from build123d import *

# Parameters (mm, degrees)
SKETCH1_R           = 1.5
BOSS_EXTRUDE1_DEPTH = 7
SKETCH2_R           = 1.4
BOSS_EXTRUDE2_DEPTH = 0.5
BOSS_EXTRUDE3_START = 0.5
SKETCH3_R           = 1.5
BOSS_EXTRUDE3_DEPTH = 0.5


with BuildPart() as part:
    # Sketch1 → Boss-Extrude1 (new body)
    with BuildSketch(Plane.XY):
        Circle(SKETCH1_R)
    extrude(amount=BOSS_EXTRUDE1_DEPTH)

    # Sketch2 → Boss-Extrude2 (add)
    with BuildSketch(Plane(origin=(0, 0, 0), x_dir=(-1, 0, 0), z_dir=(0, 0, -1))):
        Circle(SKETCH2_R)
    boss_extrude2 = extrude(amount=BOSS_EXTRUDE2_DEPTH)

    # Sketch3 → Boss-Extrude3 (add)
    with BuildSketch(Plane(origin=(0, 0, -0.5), x_dir=(-1, 0, 0), z_dir=(0, 0, -1)).offset(BOSS_EXTRUDE3_START)):
        with Locations(Location((0, 0, 0), (0, 0, 180))):
            Circle(SKETCH3_R)
    boss_extrude3 = extrude(amount=-BOSS_EXTRUDE3_DEPTH)

    # Mirror1: Boss-Extrude2, Boss-Extrude3 across plane
    add(boss_extrude2.mirror(Plane.XY.offset(3.5)))
    add(boss_extrude3.mirror(Plane.XY.offset(3.5)))


solid = part.part
Design review of the part built by this model. Coordinates are the model's own, in mm. Round coordinates to 2 decimals unless told otherwise and drop trailing zeros. Write each loop counter-clockwise with the first axis right and the second up, starting at its lowest first coordinate (ties: lowest second). Pieces come first, ordered by that corner, then holes. Notation, with made-up numbers: (-7.5, 40.25) - (28.5, 40.25) arc R23 cw to (28.5, 65.25) - close; hole circle Ø5 at (-8.5, 38). An arc over 180 degrees is marked (long way). Return JSON: item names as keys, results as strings. Group by question number.
Item 1: We need section C-C on z = 2.25. Write out the cut boundary in (x, y).
Item 2: The part is to be moulded in two halves that separate along Z. For faces 1 (the face through (1.4, 0.06, -0.25)), 2 (the face through (1.43, -0.45, -0.75)), 3 (the face through (0, 0, -1)), 4 (the face through (1.4, 0.06, 7.25)), say which applies: pulls with the +Z half, pulls with the -Z half, needs draft (parallel to the pull), parting line crosses it, or undercut.
Item 3: We need section B-B on x = 0.95. Write out the cut boundary in (y, z), and give its area (3 significant figures).
Item 4: We need section A-A on y = -0.35. Write out the cut boundary in (x, z).
Item 5: For probe 1 along X at (y, z) = (1.1, 3.5); probe 2 along X at (y, z) = (1.3, 5.5); probe 3 along Y at (x, z) = (0.15, 7.25), list the stretches that pass through material, from the lowest coordinate up. Write a range as [from, to].
Model answer:
{
 "1": {"outline": "circle Ø3 at (0, 0)"},
 "2": {"face 1": "undercut", "face 2": "needs draft", "face 3": "pulls with the -Z half", "face 4": "undercut"},
 "3": {"outline": "(-1.16, -1) - (1.16, -1) - (1.16, -0.5) - (1.03, -0.5) - (1.03, 0) - (1.16, 0) - (1.16, 7) - (1.03, 7) - (1.03, 7.5) - (1.16, 7.5) - (1.16, 8) - (-1.16, 8) - (-1.16, 7.5) - (-1.03, 7.5) - (-1.03, 7) - (-1.16, 7) - (-1.16, 0) - (-1.03, 0) - (-1.03, -0.5) - (-1.16, -0.5) - close", "area": "20.6 mm²"},
 "4": {"outline": "(-1.46, -1) - (1.46, -1) - (1.46, -0.5) - (1.36, -0.5) - (1.36, 0) - (1.46, 0) - (1.46, 7) - (1.36, 7) - (1.36, 7.5) - (1.46, 7.5) - (1.46, 8) - (-1.46, 8) - (-1.46, 7.5) - (-1.36, 7.5) - (-1.36, 7) - (-1.46, 7) - (-1.46, 0) - (-1.36, 0) - (-1.36, -0.5) - (-1.46, -0.5) - close"},
 "5": {"probe 1": "x = [-1.02, 1.02]", "probe 2": "x = [-0.75, 0.75]", "probe 3": "y = [-1.39, 1.39]"}
}
